from build123d import *

# Parameters (mm, degrees)
SKETCH1_R           = 3
BOSS_EXTRUDE1_DEPTH = 2
SKETCH2_R           = 1.5
BOSS_EXTRUDE2_DEPTH = 25
SKETCH3_W           = 0.9
SKETCH3_H           = 0.9
SKETCH3_W_2         = 1.05
SKETCH3_H_2         = 1.05
CUT_EXTRUDE1_DEPTH  = 1.9
FILLET1_R           = 0.4


with BuildPart() as part:
    # Sketch1 → Boss-Extrude1 (new body)
    with BuildSketch(Plane(origin=(0, 0, 0), x_dir=(1, 0, 0), z_dir=(0, 1, 0))):
        Circle(SKETCH1_R)
    extrude(amount=BOSS_EXTRUDE1_DEPTH)

    # Sketch2 → Boss-Extrude2 (add)
    with BuildSketch(Plane(origin=(0, 2, 0), x_dir=(1, 0, 0), z_dir=(0, 1, 0))):
        Circle(SKETCH2_R)
    extrude(amount=BOSS_EXTRUDE2_DEPTH)

    # Sketch3 → Cut-Extrude1 (cut)
    with BuildSketch(Plane(origin=(0, 0, 0), x_dir=(-1, 0, 0), z_dir=(0, -1, 0))):
        Rectangle(SKETCH3_W, SKETCH3_H)
        with Locations((0.975, 0)):
            Rectangle(SKETCH3_W_2, SKETCH3_H)
        with Locations((0, -0.975)):
            Rectangle(SKETCH3_W, SKETCH3_H_2)
        with Locations((-0.975, 0)):
            Rectangle(SKETCH3_W_2, SKETCH3_H)
        with Locations((0, 0.975)):
            Rectangle(SKETCH3_W, SKETCH3_H_2)
    extrude(amount=-CUT_EXTRUDE1_DEPTH, mode=Mode.SUBTRACT)

    # Fillet1
    fillet1_edges = [part.edges().sort_by_distance(p)[0] for p in [
        (-3, 0, 0),
        (-3, 2, 0),
    ]]
    fillet(fillet1_edges, radius=FILLET1_R)


solid = part.part
Check sheet for the modelled part. Datum: model origin and axes. Units: mm. A direction names the side the tool comes from. Round coordinates to 2 decimals unless told otherwise and drop trailing zeros. Loops run counter-clockwise (first coordinate to the right, second up) from the corner with the lowest first, then second, coordinate; pieces in that order, holes last. Notation, with made-up numbers: (-11, 85) -> (-3, 85) arc R22 ccw to (-3, 121) -> close; hole circle Ø8 at (33, 89.5). An arc over 180 degrees is marked (long way). Put each result on its own line as item: value. Start each with the question number.
1. Section check C-C (y = 13.75). Enter the section's corners in (x, z), plus the area to 3 significant figures.
2. Section check B-B (z = 0). Enter the section's corners in (x, y), plus the area to 3 significant figures.
3. Gauge pin test, flat ends, axial feed: pin 1 (0.8 mm diameter, centred on y = 0.5, z = 1, fed in from -X); pin 2 (0.5 mm diameter, centred on x = -1, y = 0.5, fed in from -Z); pin 3 (1.5 mm diameter, centred on x = -0.5, y = 24, fed in from -Z). Record the tip position at first contact, or that the pin passes through.
4. Scan lines: probe 1 along Y at (x, z) = (-1.6, -1.55); probe 2 along Z at (x, y) = (0, 15); probe 3 along X at (y, z) = (5.5, 0.2). Record each from-to range of solid material in increasing order.
5. Draft check along Z on faces 1 (the face through (-1.5, 14.32, -0.07)), 2 (the face through (0, 27, 0)), 3 (the face through (0.45, 1, 1)). Enter one of: +Z half, -Z half, draft (parallel to the pull), parting line (faces both ways), or undercut.
6. Access from +Z, -Z, +X, -X, +Y, -Y to the whole of each face (thin tool, end or side, straight path). Record for faces 4 (the face through (2, 2, 0)), 5 (the face through (1, 0, 1)), 6 (the face through (0.45, 1, -1)).
7. Section check A-A (x = 0). Enter the section's corners in (y, z).
Findings:
1. outline: circle Ø3 at (0, 0)
1. area: 7.07 mm^2
2. outline: (-3, 0.4) arc R0.4 ccw to (-2.6, 0) -> (-1.5, 0) -> (-1.5, 1.9) -> (1.5, 1.9) -> (1.5, 0) -> (2.6, 0) arc R0.4 ccw to (3, 0.4) -> (3, 1.6) arc R0.4 ccw to (2.6, 2) -> (1.5, 2) -> (1.5, 27) -> (-1.5, 27) -> (-1.5, 2) -> (-2.6, 2) arc R0.4 ccw to (-3, 1.6) -> close
2. area: 81.2 mm^2
3. pin 1: stops at x = -2.94
3. pin 2: stops at z = -2.9
3. pin 3: stops at z = -1.5
4. probe 1: y = 0 to 2
4. probe 2: z = -1.5 to 1.5
4. probe 3: x = -1.49 to 1.49
5. face 1: parting line
5. face 2: draft
5. face 3: undercut
6. face 4: +Y
6. face 5: +Z, -Z, +X, -X, -Y
6. face 6: -Y
7. outline: (0, -2.6) arc R0.4 ccw to (0.4, -3) -> (1.6, -3) arc R0.4 ccw to (2, -2.6) -> (2, -1.5) -> (27, -1.5) -> (27, 1.5) -> (2, 1.5) -> (2, 2.6) arc R0.4 ccw to (1.6, 3) -> (0.4, 3) arc R0.4 ccw to (0, 2.6) -> (0, 1.5) -> (1.9, 1.5) -> (1.9, -1.5) -> (0, -1.5) -> close
